The model under review builds one solid part; all positions refer to its coordinate system, in mm. A direction names the side the tool comes from. Coordinates: 2 decimals unless noted, no trailing zeros. Write each loop counter-clockwise with the first axis right and the second up, starting at its lowest first coordinate (ties: lowest second). Pieces come first, ordered by that corner, then holes.
1) For P1, Ø5.5, axis at y = 69.5, z = 32.5, coming from the -X side; P2, Ø18, axis at x = 49.5, y = 28, coming from the +Z side; P3, Ø5, axis at x = 1.5, y = 43.5, coming from the +Z side, all flat-tipped, find the tip position at first contact; note any pin that passes through.
2) Add section D-D, the plane z = 51. State the section outline as (x, y) points (3 decimals).
3) For line 1 (Y direction, x = 48.5, z = -11) (3 decimals); line 2 (Z direction, x = 83, y = 92); line 3 (Y direction, x = 49, z = 48) (3 decimals), list the stretches that pass through material, from the lowest coordinate up.
4) Add section B-B, the plane z = 22. Give the number of separate pieces and of enclosed holes in the cut face, then the cut area to 3 significant figures.
5) Mouldability with a two-part tool opening along Z and no side actions: class faces 1 (the cylindrical face through (-38.097, 66.586, 43.142)), 2 (the flat face through (-120.65, 67, 32)), 3 (the cylindrical face through (-80, 66.6, 48.9)) as released by +Z, released by -Z, zero draft, split by the parting line, or undercut.
6) Machinability: for faces 4 (the flat face through (0, 67, 55.562)), 5 (the flat face through (-120.65, 103, 4)), 6 (the flat face through (2, 63, -26.988)), which of the approach directions +Z, -Z, +X, -X, +Y, -Y give a long, thin tool a straight path to every point of the face, cutting with its end or side? Answer none if there is none.
from build123d import *

# Parameters (mm, degrees)
F0_W      = 260.35
F0_H      = 53.975
F1_DEPTH  = 9.525
F2_W      = 9.525
F2_H      = 53.975
F3_DEPTH  = 133.35
F4_W      = 260.3500093699
F4_H      = 53.975061956
F5_DEPTH  = 9.525
F6_W      = 260.3500093699
F6_H      = 9.525
F7_DEPTH  = 152.4
F8_W      = 241.3
F8_H      = 12.7
F9_DEPTH  = 88.9
F11_DEPTH = 12.7
F13_DEPTH = 102.108
F14_W     = 9.525
F14_H     = 60.325
F15_DEPTH = 44.45
F16_W     = 9.525
F16_H     = 60.325
F17_DEPTH = 44.45


with BuildPart() as f1:
    # F0 (on Front) → F1 (new body)
    with BuildSketch(Plane.XZ):
        Rectangle(F0_W, F0_H)
    extrude(amount=F1_DEPTH)

    # F2 (on face) → F3 (join)
    with BuildSketch(Plane(origin=(0, 0, 0), x_dir=(-1, 0, 0), z_dir=(0, 1, 0))):
        with Locations((-125.4125, 0)):
            Rectangle(F2_W, F2_H)
        with Locations((125.4125, 0)):
            Rectangle(F2_W, F2_H)
    extrude(amount=F3_DEPTH)

    # F4 (on face) → F5 (join)
    with BuildSketch(Plane(origin=(0, 133.35, 0), x_dir=(-1, 0, 0), z_dir=(0, 1, 0))):
        with Locations((4.6849e-06, -3.0978e-05)):
            Rectangle(F4_W, F4_H)
    extrude(amount=F5_DEPTH)

    # F6 (on face) → F7 (join)
    with BuildSketch(Plane(origin=(0, 142.875, 0), x_dir=(-1, 0, 0), z_dir=(0, 1, 0))):
        with Locations((4.6849e-06, -22.225030978)):
            Rectangle(F6_W, F6_H)
    extrude(amount=-F7_DEPTH)

    # F8 (on face) → F9 (join)
    with BuildSketch(Plane.XY.offset(-17.462530978)):
        with Locations((0, 66.675)):
            Rectangle(F8_W, F8_H)
    extrude(amount=F9_DEPTH)

    # F10 (on face) → F11 (cut)
    with BuildSketch(Plane.XZ.offset(-60.325)):
        with BuildLine():
            Line((25.4, 55.562469022), (-25.4, 55.562469022))
            ThreePointArc((-25.4, 55.562469022), (-38.1, 42.862469022), (-25.4, 30.162469022))
            Line((-25.4, 30.162469022), (25.4, 30.162469022))
            ThreePointArc((25.4, 30.162469022), (38.1, 42.862469022), (25.4, 55.562469022))
        make_face()
    extrude(amount=-F11_DEPTH, mode=Mode.SUBTRACT)

    # F12 (on Front) → F13 (cut)
    with BuildSketch(Plane.XZ):
        with BuildLine():
            ThreePointArc((0, 129.1245525755), (-12.2174, 188.9125), (0, 248.7004474245))
            ThreePointArc((0, 248.7004474245), (-292.5826, 188.9125), (0, 129.1245525755))
        make_face()
        with BuildLine():
            ThreePointArc((0, 248.7004474245), (9.1318136378, 219.4242334807), (12.2174, 188.9125))
            ThreePointArc((12.2174, 188.9125), (9.1318136378, 158.4007665193), (0, 129.1245525755))
            ThreePointArc((0, 129.1245525755), (170.6943334807, 39.5980863622), (292.5826, 188.9125))
            ThreePointArc((292.5826, 188.9125), (170.6943334807, 338.2269136378), (0, 248.7004474245))
        make_face()
    extrude(amount=-F13_DEPTH, mode=Mode.SUBTRACT)

    # F14 (on face) → F15 (join)
    with BuildSketch(Plane.XY.offset(-17.462530978)):
        with Locations((0, 103.1875)):
            Rectangle(F14_W, F14_H)
    extrude(amount=F15_DEPTH)

    # F16 (on face) → F17 (join)
    with BuildSketch(Plane.XY.offset(-17.462530978)):
        with Locations((0, 30.1625)):
            Rectangle(F16_W, F16_H)
    extrude(amount=F17_DEPTH)


solid = f1.part
Geometry results:
1. P1: stops at x = -120.65
1. P2: stops at z = -17.46
1. P3: stops at z = 26.99
2. outline: (-75.33, 60.325) - (-35.15, 60.325) - (-35.15, 73.025) - (-75.33, 73.025) - close; (35.15, 60.325) - (75.33, 60.325) - (75.33, 73.025) - (35.15, 73.025) - close
3. line 1: y = -9.525 to 0, 60.325 to 73.025, 133.35 to 142.875
3. line 2: z = -26.99 to -17.46
3. line 3: y = 60.325 to 73.025
4. separate pieces: 1
4. enclosed holes: 4
4. area: 11,700 mm2
5. face 1: undercut
5. face 2: zero draft
5. face 3: released by +Z
6. face 4: +Y, -Y
6. face 5: +Z
6. face 6: -Z, +X, -X, +Y, -Y
